For this review, take the finished solid that the model builds, in its own axes (mm). A direction names the side the tool comes from. Give positions to 0.01 mm unless a question says otherwise; leave off trailing zeros. Loops run counter-clockwise (first coordinate to the right, second up) from the corner with the lowest first, then second, coordinate; pieces in that order, holes last. Notation, with made-up numbers: (1, -16) - (14, -16) arc R20 ccw to (14, 18) - close; hole circle Ø4 at (2, 12). An arc over 180 degrees is marked (long way). Answer in a Markdown table with one row per item.
```python
from build123d import *

# Parameters (mm, degrees)
SKETCH2_W           = 131.7
SKETCH2_H           = 62.2
BOSS_EXTRUDE1_DEPTH = 14.7
SKETCH3_W           = 127.9
SKETCH3_H           = 58.4
CUT_EXTRUDE1_DEPTH  = 13
SKETCH4_W           = 20.3
SKETCH4_H           = 9.9
BOSS_EXTRUDE2_DEPTH = 2.2
FILLET1_R           = 3
SKETCH5_W           = 1.5
SKETCH5_H           = 2
SKETCH5_W_2         = 2
BOSS_EXTRUDE3_DEPTH = 2
CUT_EXTRUDE2_DEPTH  = 200


with BuildPart() as part:
    # Sketch2 → Boss-Extrude1 (new body)
    with BuildSketch(Plane(origin=(0, 0, 0), x_dir=(1, 0, 0), z_dir=(0, 1, 0))):
        Rectangle(SKETCH2_W, SKETCH2_H)
    extrude(amount=BOSS_EXTRUDE1_DEPTH)

    # Sketch3 → Cut-Extrude1 (cut)
    with BuildSketch(Plane(origin=(0, 14.7, 0), x_dir=(1, 0, 0), z_dir=(0, 1, 0))):
        Rectangle(SKETCH3_W, SKETCH3_H)
    extrude(amount=-CUT_EXTRUDE1_DEPTH, mode=Mode.SUBTRACT)

    # Sketch4 → Boss-Extrude2 (add)
    with BuildSketch(Plane.XZ):
        with Locations((0, 36.05)):
            Rectangle(SKETCH4_W, SKETCH4_H)
    extrude(amount=-BOSS_EXTRUDE2_DEPTH)

    # Fillet1
    fillet1_edges = [part.edges().sort_by_distance(p)[0] for p in [
        (-10.15, 1.1, 41),
        (10.15, 1.1, 41),
    ]]
    fillet(fillet1_edges, radius=FILLET1_R)

    # Sketch5 → Boss-Extrude3 (add)
    with BuildSketch(Plane.XY.offset(31.1)):
        with Locations((-65.1, 7.35)):
            Rectangle(SKETCH5_W, SKETCH5_H)
        with Locations((-66.85, 7.35)):
            Rectangle(SKETCH5_W_2, SKETCH5_H)
        Polygon((-65.85, 4.35), (-65.85, 6.35), (-67.85, 6.35), align=None)
        Polygon((-64.35, 6.35), (-65.85, 6.35), (-65.85, 4.35), (-64.35, 2.85), align=None)
    boss_extrude3 = extrude(amount=BOSS_EXTRUDE3_DEPTH)

    # Mirror1: Boss-Extrude3 across plane
    add(boss_extrude3.mirror(Plane(origin=(0, 0, 0), x_dir=(0, 0, 1), z_dir=(1, 0, 0))))

    # Sketch6 → Cut-Extrude2 (cut, symmetric)
    with BuildSketch(Plane.ZY.offset(65.85)):
        Polygon((33.1, 6.35), (31.1, 2.85), (33.1, 2.85), align=None)
    extrude(amount=CUT_EXTRUDE2_DEPTH, both=True, mode=Mode.SUBTRACT)


solid = part.part
```
1. We need section A-A, the plane y = 13.25. Give the boundary of the cut face in (x, z).
Values:
| item | result |
|---|---|
| outline | (-65.85, -31.1) - (65.85, -31.1) - (65.85, 31.1) - (-65.85, 31.1) - close; hole (-63.95, -29.2) - (63.95, -29.2) - (63.95, 29.2) - (-63.95, 29.2) - close |
2. We need section B-B, the plane x = -4.5. Give the boundary of the cut face in (y, z), and give its area (3 significant figures).
Values:
| item | result |
|---|---|
| outline | (0, -31.1) - (14.7, -31.1) - (14.7, -29.2) - (1.7, -29.2) - (1.7, 29.2) - (14.7, 29.2) - (14.7, 31.1) - (2.2, 31.1) - (2.2, 41) - (0, 41) - close |
| area | 177 mm^2 |
3. Wall thickness on line 1 (X direction, y = 3.5, z = -16); line 2 (Z direction, x = -51, y = 6); line 3 (X direction, y = 6.75, z = 32): over which ranges is each line inside the solid? List them lowest first. Write a range as [from, to].
Values:
| item | result |
|---|---|
| line 1 | x = [-65.85, -63.95], [63.95, 65.85] |
| line 2 | z = [-31.1, -29.2], [29.2, 31.1] |
| line 3 | x = [-67.85, -64.35], [64.35, 67.85] |
4. Clearance check with flat-ended pins moving along their axes: pin 1 (0.6 mm diameter, centred on x = 65.5, y = 7.5, fed in from +Z); pin 2 (5 mm diameter, centred on x = -18.5, y = 4.5, fed in from +Z); pin 3 (2 mm diameter, centred on y = 12, z = 18.5, fed in from +X). State where each tip first meets the part, or that it passes through.
Values:
| item | result |
|---|---|
| pin 1 | stops at z = 33.1 |
| pin 2 | stops at z = 31.1 |
| pin 3 | stops at x = 65.85 |
5. We need section D-D, the plane x = 51.5. Give the boundary of the cut face in (y, z), and give its area (3 significant figures).
Values:
| item | result |
|---|---|
| outline | (0, -31.1) - (14.7, -31.1) - (14.7, -29.2) - (1.7, -29.2) - (1.7, 29.2) - (14.7, 29.2) - (14.7, 31.1) - (0, 31.1) - close |
| area | 155 mm^2 |
6. We need section C-C, the plane z = 11.5. Give the boundary of the cut face in (x, y), and give its area (3 significant figures).
Values:
| item | result |
|---|---|
| outline | (-65.85, 0) - (65.85, 0) - (65.85, 14.7) - (63.95, 14.7) - (63.95, 1.7) - (-63.95, 1.7) - (-63.95, 14.7) - (-65.85, 14.7) - close |
| area | 273 mm^2 |
7. For faces 4 (the face through (-66.5, 5, 31.9)), 5 (the face through (-63.95, 8, 0)), 6 (the face through (0, 2.2, 36)), list the 3-axis set-ups (+Z, -Z, +X, -X, +Y, -Y) from which the entire face can be reached by the end or side of a thin tool; tool diameter is ignored.
Values:
| item | result |
|---|---|
| face 4 | +Z, -X, -Y |
| face 5 | +Y |
| face 6 | +Z, +X, -X, +Y |
8. Mouldability with a two-part tool opening along X and no side actions: class faces 1 (the face through (66.5, 5, 31.9)), 2 (the face through (63.95, 8, 0)), 3 (the face through (-65.85, 7, 0)) as released by +X, released by -X, zero draft, split by the parting line, or undercut.
Values:
| item | result |
|---|---|
| face 1 | released by +X |
| face 2 | undercut |
| face 3 | released by -X |
